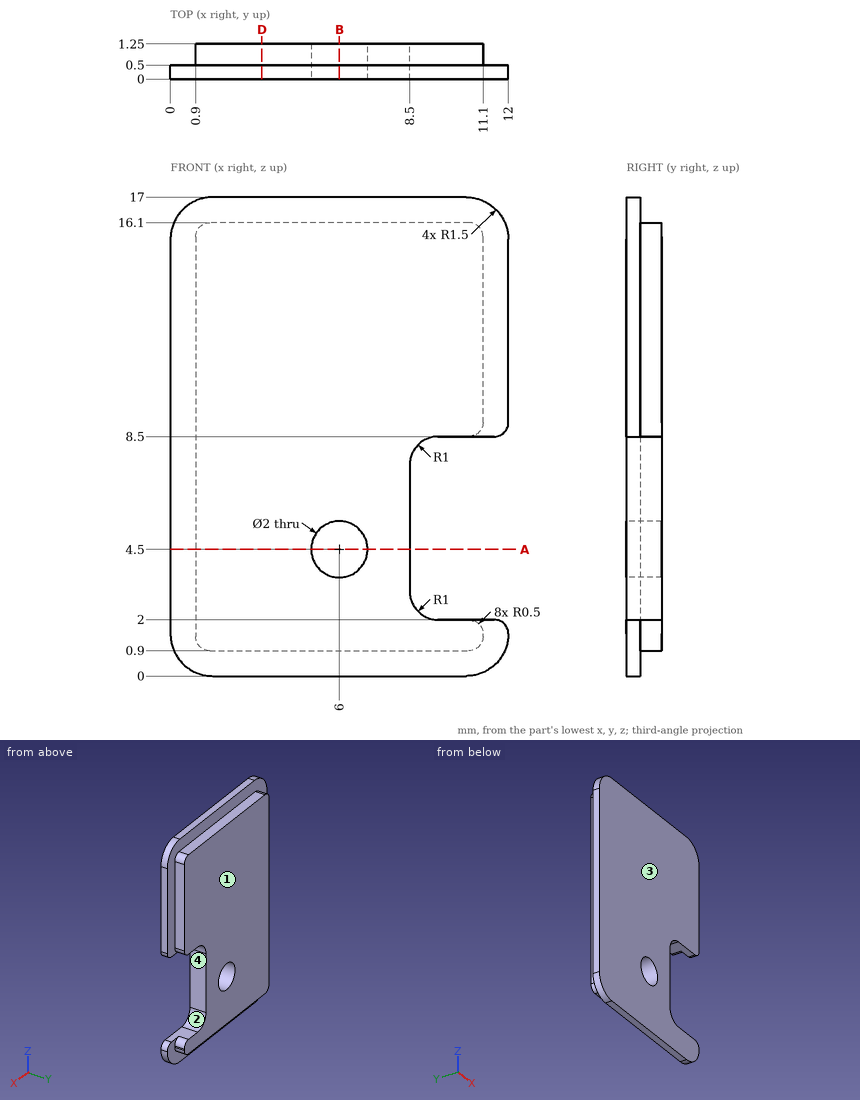
Check sheet for the drawn part. Datum: minimum x, y, z corner. Units: mm. A direction names the side the tool comes from. Coordinates: 2 decimals unless noted, no trailing zeros. Order: outer loops, then holes, each group sorted by start corner. A loop starts at its lowest first (then second) coordinate and runs counter-clockwise, first axis right, second up. Notation, with made-up numbers: M -6.5,-3.5 L 33.5,-3.5 A18 ccw 33.5,14.5 Z; hole C 36.25,-34 d6. An arc over 180 degrees is marked long. One line per question, with ' | ' between items. Start each with the question number.
Item 1: Draft check along Z on the marked faces 1 and 2. Enter one of: pulls with the +Z half, pulls with the -Z half, needs draft (parallel to the pull), parting line crosses it, or undercut.
Item 2: Cross-section at B-B on x = 6. Enter the section's corners in (y, z), then the cut area to 3 significant figures.
Item 3: Cross-section at D-D on x = 3.25. Enter the section's corners in (y, z), then the cut area to 3 significant figures.
Item 4: Set-up check for the marked faces 3 and 4: record each of +Z, -Z, +X, -X, +Y, -Y from which the full face is reachable in a straight line by a thin tool's end or side.
Item 5: Material ranges on L1, parallel to Z at x = 6, y = 0.6; L2, parallel to Z at x = 9.5, y = 0.6; L3, parallel to X at y = 1.1, z = 10.5, recorded low to high. Write a range as [from, to].
Item 6: Gauge pin test, flat ends, axial feed: pin 1 (0.6 mm diameter, centred on x = 11, y = 0.5, fed in from -Z); pin 2 (1.6 mm diameter, centred on x = 6, z = 4.5, fed in from +Y). Record the tip position at first contact, or that the pin passes through.
Item 7: Cross-section at A-A on z = 4.5. Enter the section's corners in (x, y).
Findings:
1) face 1: needs draft | face 2: undercut
2) outline: M 0,0 L 0.5,0 L 0.5,0.9 L 1.25,0.9 L 1.25,3.5 L 0,3.5 Z; M 0,5.5 L 1.25,5.5 L 1.25,16.1 L 0.5,16.1 L 0.5,17 L 0,17 Z | area: 17.4 mm²
3) outline: M 0,0 L 0.5,0 L 0.5,0.9 L 1.25,0.9 L 1.25,16.1 L 0.5,16.1 L 0.5,17 L 0,17 Z | area: 19.9 mm²
4) face 3: +Z, -Z, +X, -X, -Y | face 4: +X, +Y, -Y
5) L1: z = [0.9, 3.5], [5.5, 16.1] | L2: z = [0.9, 2], [8.5, 16.1] | L3: x = [0.9, 11.1]
6) pin 1: stops at z = 0.01 | pin 2: passes through
7) outline: M 0,0 L 5,0 L 5,1.25 L 0.9,1.25 L 0.9,0.5 L 0,0.5 Z; M 7,0 L 8.5,0 L 8.5,1.25 L 7,1.25 Z
